Input: part model. Units: mm. Frame: model coordinates. Face numbers are marked on the shaded views. A direction names the side the tool comes from. Coordinates: 2 decimals unless noted, no trailing zeros. Write each loop counter-clockwise with the first axis right and the second up, starting at its lowest first coordinate (ties: lowest second). Pieces come first, ordered by that corner, then holes. Notation, with made-up numbers: M 45,67 L 67,67 A37 ccw 67,104 Z; hole C -4.5,-12.5 d3. An arc over 180 degrees is marked long. Write each question's results on one line, items separated by ' | '. Start each with the question number.
1. First-contact query: pin 1 (1 mm diameter, centred on y = -16.5, z = 7.5, fed in from -X); pin 2 (3 mm diameter, centred on x = -15.5, z = 1.5, fed in from -Y); pin 3 (6 mm diameter, centred on x = 18, y = 10, fed in from -Z). Flat tips, straight axial feed; report the tip coordinate or a pass-through.
2. Pull-direction query (Y, two-part tool) for the marked faces 1, 2 and 3; classes: +Y half, -Y half, draft (parallel to the pull), parting line (faces both ways), or undercut.
3. Section query B-B, the plane x = 11.5. Output: boundary loops of the cut face in (y, z) (3 decimals).
4. Set-up query: the marked faces 4, 5, 6 and 7. Return all of +Z, -Z, +X, -X, +Y, -Y with unobstructed straight access to the full face (end or side cutting, diameter ignored); none if empty.
5. Section query A-A, the plane z = 0. Count the separate pieces of the cut face and the enclosed holes in it, and give its area (3 significant figures).
6. Ray query, probe 1 along Y at (x, z) = (21.5, 0) (3 decimals); probe 2 along X at (y, z) = (5.5, 0). Return the intervals inside material, ascending.
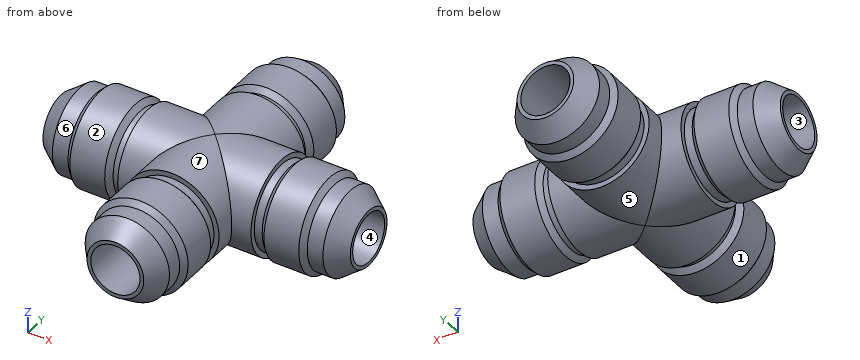
```python
from build123d import *

# Parameters (mm, degrees)
SKETCH2_R           = 9.525
EXTRUDE1_DEPTH      = 17.526
SKETCH15_R          = 9.525
BOSS_EXTRUDE1_DEPTH = 13.4239
SKETCH16_R          = 4.9657
CUT_EXTRUDE1_DEPTH  = 31.9499
CIRPATTERN1_COUNT   = 4
CIRPATTERN1_ANGLE   = 270
SKETCH17_R          = 4.9657
CUT_EXTRUDE2_DEPTH  = 62.8998
CUT_EXTRUDE3_REACH  = 63.9
SKETCH18_R          = 4.9657


with BuildPart() as part:
    # Sketch2 → Extrude1 (new body)
    with BuildSketch(Plane(origin=(-30.9499, 0, 0), x_dir=(0, 0, -1), z_dir=(1, 0, 0))):
        Circle(SKETCH2_R)
    extrude(amount=EXTRUDE1_DEPTH)

    # Sketch5 → Cut-Revolve1 (revolve, cut)
    with BuildSketch(Plane.XY):
        Polygon((-27.256291687, 8.493888504), (-24.081291687, 8.493888504), (-23.050180191, 9.525), (-30.9499, 9.525), (-30.9499, 5.710555), align=None)
        Polygon((-13.4239, 8.493888504), (-15.0114, 8.493888504), (-16.042511496, 9.525), (-13.4239, 9.525), align=None)
    revolve(axis=Axis((0, 0, 0), (-1, 0, 0)), mode=Mode.SUBTRACT)

    # Sketch15 → Boss-Extrude1 (add)
    with BuildSketch(Plane(origin=(-13.4239, 0, 0), x_dir=(0, 0, -1), z_dir=(1, 0, 0))):
        Circle(SKETCH15_R)
    extrude(amount=BOSS_EXTRUDE1_DEPTH)

    # Sketch16 → Cut-Extrude1 (cut, through all)
    with BuildSketch(Plane(origin=(0, 0, 0), x_dir=(0, 0, -1), z_dir=(1, 0, 0))):
        Circle(SKETCH16_R)
    extrude(amount=-CUT_EXTRUDE1_DEPTH, mode=Mode.SUBTRACT)


with BuildPart() as cirpattern1_1:
    # CirPattern1: pattern copy
    add(part.part.rotate(Axis((0, 0, 0), (0, 0, -1)), 1 * CIRPATTERN1_ANGLE / (CIRPATTERN1_COUNT - 1)))

    # Sketch17 → Cut-Extrude2 (cut, through all)
    with BuildSketch(Plane.ZY.offset(30.9499)):
        Circle(SKETCH17_R)
    extrude(amount=-CUT_EXTRUDE2_DEPTH, mode=Mode.SUBTRACT)


with BuildPart() as cirpattern1_2:
    # CirPattern1: pattern copy
    add(part.part.rotate(Axis((0, 0, 0), (0, 0, -1)), 2 * CIRPATTERN1_ANGLE / (CIRPATTERN1_COUNT - 1)))


with BuildPart() as cirpattern1_3:
    # CirPattern1: pattern copy
    add(part.part.rotate(Axis((0, 0, 0), (0, 0, -1)), 3 * CIRPATTERN1_ANGLE / (CIRPATTERN1_COUNT - 1)))


with BuildPart() as cirpattern1_1_1:
    add(cirpattern1_1.part)

    # Combine1: union part, CirPattern1_2, CirPattern1_3
    add(part.part)
    add(cirpattern1_2.part)
    add(cirpattern1_3.part)

    # Sketch18 → Cut-Extrude3 (cut, up to next)
    with BuildSketch(Plane(origin=(0, 30.9499, 0), x_dir=(1, 0, 0), z_dir=(0, 1, 0)), mode=Mode.PRIVATE) as cut_extrude3_sk1:
        Circle(SKETCH18_R)
    cut_extrude3_tool1 = extrude(cut_extrude3_sk1.sketch, amount=-CUT_EXTRUDE3_REACH, mode=Mode.PRIVATE) & cirpattern1_1_1.part
    add(cut_extrude3_tool1.solids().sort_by_distance((0, 30.9499, 0))[0], mode=Mode.SUBTRACT)


solid = cirpattern1_1_1.part
```
Answer:
1) pin 1: x = -6.46 | pin 2: y = -9.52 | pin 3: z = -6.46
2) face 1: draft | face 2: parting line | face 3: undercut
3) outline: C 0,0 d19.05; hole C 0,0 d9.931
4) face 4: +X | face 5: +Y | face 6: -X | face 7: -Y
5) separate pieces: 3 | enclosed holes: 0 | area: 836 mm^2
6) probe 1: -9.525 to -4.966, 4.966 to 9.525 | probe 2: -30.95 to -4.97, 4.97 to 30.95
